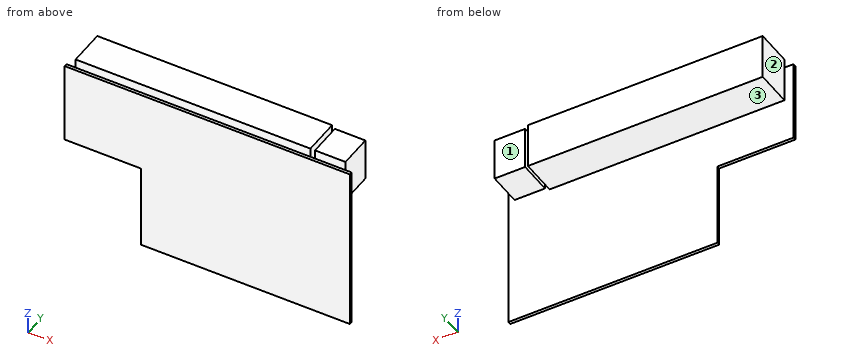
```python
from build123d import *

# Parameters (mm, degrees)
BOSS_EXTRUDE1_DEPTH = 1
SKETCH2_W           = 77
SKETCH2_H           = 15
BOSS_EXTRUDE2_DEPTH = 12
SKETCH3_W           = 10
SKETCH3_H           = 14
BOSS_EXTRUDE3_DEPTH = 11


with BuildPart() as part:
    # Sketch1 → Boss-Extrude1 (new body)
    with BuildSketch(Plane(origin=(0, 0, 0), x_dir=(1, 0, 0), z_dir=(0, 1, 0))):
        Polygon((-46.9670263, -0.627662529), (-21.9670263, -0.627662529), (-21.9670263, 27.372337471), (46.5329737, 27.372337471), (46.5329737, -27.627662529), (-46.9670263, -27.627662529), align=None)
    extrude(amount=BOSS_EXTRUDE1_DEPTH)

    # Sketch2 → Boss-Extrude2 (add)
    with BuildSketch(Plane(origin=(0, 1, 0), x_dir=(1, 0, 0), z_dir=(0, 1, 0))):
        with Locations((-5.4670263, -23.127662529)):
            Rectangle(SKETCH2_W, SKETCH2_H)
    extrude(amount=BOSS_EXTRUDE2_DEPTH)

    # Sketch3 → Boss-Extrude3 (add)
    with BuildSketch(Plane(origin=(0, 1, 0), x_dir=(1, 0, 0), z_dir=(0, 1, 0))):
        with Locations((39.5329737, -23.627662529)):
            Rectangle(SKETCH3_W, SKETCH3_H)
    extrude(amount=BOSS_EXTRUDE3_DEPTH)


solid = part.part
```
Here's how the part is built. I have some questions about the finished solid (model axes, mm). Face numbers are marked on the shaded views. A direction names the side the tool comes from. Round coordinates to 2 decimals unless told otherwise and drop trailing zeros. Write each loop counter-clockwise with the first axis right and the second up, starting at its lowest first coordinate (ties: lowest second). Pieces come first, ordered by that corner, then holes.
Q1. Which directions (+Z, -Z, +X, -X, +Y, -Y) give clear straight access to the entire face, cutting with the end or side of a thin tool? Please do the marked faces 1, 2 and 3.
Q2. If we section it at A-A on y = 7.75: Write out the boundary of the cut face in (x, z), plus the area to 4 significant figures.
Q3. Please list where these lines run through material, in increasing order: probe 1 along X at (y, z) = (8, 28); probe 2 along Z at (x, y) = (13.5, 1.75); probe 3 along Y at (x, z) = (23, 3).
Q4. If we section it at B-B on x = 21: Write out the boundary of the cut face in (y, z).
Q5. If we section it at C-C on z = 21.5: Write out the boundary of the cut face in (x, y), plus the area to 3 significant figures.
Q6. Will these pins go through, and if not, where does the flat tip stop? P1, Ø0.5, axis at x = -40, y = 0.5, coming from the -Z side; P2, Ø1.5, axis at y = 3, z = 8, coming from the +X side; P3, Ø5.5, axis at y = 8.5, z = 27, coming from the +X side; P4, Ø1.5, axis at x = 1.5, z = 28.5, coming from the -Y side.
Q7. If we section it at D-D on x = 40.5: Write out the boundary of the cut face in (y, z).
Answer below:
1. face 1: +Z, -Z, +X, +Y
1. face 2: +Z, -Z, -X, +Y
1. face 3: -Z, +X, -X, +Y
2. outline: (-43.97, 15.63) - (33.03, 15.63) - (33.03, 30.63) - (-43.97, 30.63) - close; (34.53, 16.63) - (44.53, 16.63) - (44.53, 30.63) - (34.53, 30.63) - close
2. area: 1,295 mm2
3. probe 1: x = -43.97 to 33.03, 34.53 to 44.53
3. probe 2: z = 15.63 to 30.63
3. probe 3: y = 0 to 1
4. outline: (0, -27.37) - (1, -27.37) - (1, 15.63) - (13, 15.63) - (13, 30.63) - (1, 30.63) - (1, 27.63) - (0, 27.63) - close
5. outline: (-46.97, 0) - (46.53, 0) - (46.53, 1) - (44.53, 1) - (44.53, 12) - (34.53, 12) - (34.53, 1) - (33.03, 1) - (33.03, 13) - (-43.97, 13) - (-43.97, 1) - (-46.97, 1) - close
5. area: 1,130 mm2
6. P1: stops at z = 0.63
6. P2: passes through
6. P3: stops at x = 44.53
6. P4: stops at y = 1
7. outline: (0, -27.37) - (1, -27.37) - (1, 16.63) - (12, 16.63) - (12, 30.63) - (1, 30.63) - (1, 27.63) - (0, 27.63) - close
